For this review, take the finished solid that the model builds, in its own axes (mm). A direction names the side the tool comes from. Give positions to 0.01 mm unless a question says otherwise; leave off trailing zeros. Loops run counter-clockwise (first coordinate to the right, second up) from the corner with the lowest first, then second, coordinate; pieces in that order, holes last. Notation, with made-up numbers: (66.25, 74) - (111.25, 74) arc R15 cw to (111.25, 91) - close; hole circle Ø11 at (88.25, -16.5). An arc over 180 degrees is marked (long way). Put each result on its own line as item: value.
from build123d import *

# Parameters (mm, degrees)
BOSS_EXTRUDE1_DEPTH     = 381
SKETCH2_R               = 3.175
CUT_EXTRUDE1_DEPTH      = 1
CUT_EXTRUDE1_DEPTH_BACK = 64.5
CUT_EXTRUDE3_DEPTH      = 12.7
SKETCH7_R               = 14.2875
CUT_EXTRUDE4_DEPTH      = 14.97
CUT_EXTRUDE4_DEPTH_BACK = 50.53
SKETCH8_R               = 3.175
CUT_EXTRUDE5_DEPTH      = 1
CUT_EXTRUDE5_DEPTH_BACK = 64.5
SKETCH9_R               = 14.2875
CUT_EXTRUDE6_DEPTH      = 152.4


with BuildPart() as part:
    # Sketch1 → Boss-Extrude1 (new body)
    with BuildSketch(Plane.XY):
        Polygon((0, 0), (63.5, 0), (63.5, 63.5), (60.325, 63.5), (60.325, 3.175), (3.175, 3.175), (3.175, 63.5), (0, 63.5), align=None)
    extrude(amount=BOSS_EXTRUDE1_DEPTH)

    # Sketch2 → Cut-Extrude1 (cut, two sides)
    with BuildSketch(Plane.XZ) as cut_extrude1_sk:
        with Locations((12.7, 361.95)):
            Circle(SKETCH2_R)
        with Locations((50.8, 361.95)):
            Circle(SKETCH2_R)
        with Locations((12.7, 57.15)):
            Circle(SKETCH2_R)
        with Locations((12.7, 133.35)):
            Circle(SKETCH2_R)
        with Locations((12.7, 209.55)):
            Circle(SKETCH2_R)
    extrude(amount=CUT_EXTRUDE1_DEPTH, mode=Mode.SUBTRACT)
    extrude(cut_extrude1_sk.sketch, amount=-CUT_EXTRUDE1_DEPTH_BACK, mode=Mode.SUBTRACT)

    # Sketch4 → Cut-Extrude3 (cut)
    with BuildSketch(Plane.XZ):
        with BuildLine():
            Line((24.13, 323.85), (24.13, 285.75))
            ThreePointArc((24.13, 285.75), (13.97, 275.59), (3.81, 285.75))
            Line((3.81, 285.75), (3.81, 323.85))
            ThreePointArc((3.81, 323.85), (13.97, 334.01), (24.13, 323.85))
        make_face()
    extrude(amount=-CUT_EXTRUDE3_DEPTH, mode=Mode.SUBTRACT)

    # Sketch7 → Cut-Extrude4 (cut, two sides)
    with BuildSketch(Plane.ZY.offset(-13.97)) as cut_extrude4_sk:
        with Locations((304.8, 38.1)):
            Circle(SKETCH7_R)
    extrude(amount=CUT_EXTRUDE4_DEPTH, mode=Mode.SUBTRACT)
    extrude(cut_extrude4_sk.sketch, amount=-CUT_EXTRUDE4_DEPTH_BACK, mode=Mode.SUBTRACT)

    # Sketch8 → Cut-Extrude5 (cut, two sides)
    with BuildSketch(Plane.XZ) as cut_extrude5_sk:
        with Locations((38.735, 304.8)):
            Circle(SKETCH8_R)
        with Locations((53.975, 316.23)):
            Circle(SKETCH8_R)
        with Locations((53.975, 293.37)):
            Circle(SKETCH8_R)
    extrude(amount=CUT_EXTRUDE5_DEPTH, mode=Mode.SUBTRACT)
    extrude(cut_extrude5_sk.sketch, amount=-CUT_EXTRUDE5_DEPTH_BACK, mode=Mode.SUBTRACT)

    # Sketch9 → Cut-Extrude6 (cut)
    with BuildSketch(Plane.ZY):
        with Locations((25.4, 38.1)):
            Circle(SKETCH9_R)
    extrude(amount=-CUT_EXTRUDE6_DEPTH, mode=Mode.SUBTRACT)


solid = part.part
1) Take a section at A-A on z = 304.8. State the section outline as (x, y) points (1 decimal), and give its area (3 significant figures).
Geometry check:
outline: (0, 0) - (3.8, 0) - (3.8, 3.2) - (3.2, 3.2) - (3.2, 23.8) - (0, 23.8) - close; (0, 52.4) - (3.2, 52.4) - (3.2, 63.5) - (0, 63.5) - close; (24.1, 0) - (35.6, 0) - (35.6, 3.2) - (24.1, 3.2) - close; (41.9, 0) - (63.5, 0) - (63.5, 23.8) - (60.3, 23.8) - (60.3, 3.2) - (41.9, 3.2) - close; (60.3, 52.4) - (63.5, 52.4) - (63.5, 63.5) - (60.3, 63.5) - close
area: 319 mm²
2) Draft analysis for pull direction X (two halves, no side actions). For faces 4 (the face through (63.5, 31, 188)), 5 (the face through (0, 32, 188)), 6 (the face through (12.3, 1.6, 365.1)), 7 (the face through (1.61, 42.39, 318.43)), state which applies: pulls with the +X half, pulls with the -X half, needs draft (parallel to the pull), parting line crosses it, or undercut.
Geometry check:
face 4: pulls with the +X half
face 5: pulls with the -X half
face 6: undercut
face 7: needs draft
3) Wall thickness on line 1 (Z direction, x = 1, y = 38); line 2 (X direction, y = 0.9, z = 293.37); line 3 (Y direction, x = 61.3, z = 25.4): over which ranges is each line inside the solid? List them lowest first.
Geometry check:
line 1: z = 0 to 11.11, 39.69 to 290.51, 319.09 to 381
line 2: x = 0 to 3.81, 24.13 to 50.8, 57.15 to 63.5
line 3: y = 0 to 23.81, 52.39 to 63.5
4) Take a section at B-B on y = 16. State the section outline as (x, z) points (3 decimals), and give its area (3 significant figures).
Geometry check:
outline: (0, 0) - (3.175, 0) - (3.175, 381) - (0, 381) - close; (60.325, 0) - (63.5, 0) - (63.5, 381) - (60.325, 381) - close
area: 2,420 mm²
5) Take a section at D-D on x = 12.7. State the section outline as (y, z) points (3 decimals), and give its area (3 significant figures).
Geometry check:
outline: (0, 0) - (3.175, 0) - (3.175, 53.975) - (0, 53.975) - close; (0, 60.325) - (3.175, 60.325) - (3.175, 130.175) - (0, 130.175) - close; (0, 136.525) - (3.175, 136.525) - (3.175, 206.375) - (0, 206.375) - close; (0, 212.725) - (3.175, 212.725) - (3.175, 275.67) - (0, 275.67) - close; (0, 333.93) - (3.175, 333.93) - (3.175, 358.775) - (0, 358.775) - close; (0, 365.125) - (3.175, 365.125) - (3.175, 381) - (0, 381) - close
area: 944 mm²
6) Take a section at C-C on z = 209.55. State the section outline as (x, y) points (3 decimals).
Geometry check:
outline: (0, 0) - (9.525, 0) - (9.525, 3.175) - (3.175, 3.175) - (3.175, 63.5) - (0, 63.5) - close; (15.875, 0) - (63.5, 0) - (63.5, 63.5) - (60.325, 63.5) - (60.325, 3.175) - (15.875, 3.175) - close
7) Insertion check: pin 1 Ø10 at (x, z) = (38.735, 304.8) entering from +Y (3 decimals). The pin has a flat end and moves straight along its axis. Give the tip position at first contact, or say it passes through.
Geometry check:
pin 1: stops at y = 3.175
8) For faces 1 (the face through (61.89, 42.39, 318.43)), 2 (the face through (14.193, 1.565, 275.592)), 3 (the face through (3.175, 33, 188)), list the 3-axis set-ups (+Z, -Z, +X, -X, +Y, -Y) from which the entire face can be reached by the end or side of a thin tool; tool diameter is ignored.
Geometry check:
face 1: +X, -X
face 2: +Y, -Y
face 3: +Z, -Z, +Y
